```python
from build123d import *

# Parameters (mm, degrees)
BOSS_EXTRUDE1_DEPTH   = 50
BOSS_EXTRUDE1_2_DEPTH = 50
SKETCH3_W             = 160
SKETCH3_H             = 200
BOSS_EXTRUDE2_DEPTH   = 10
FILLET1_R             = 5


with BuildPart() as part:
    # Sketch2 → Boss-Extrude1 (new body)
    with BuildSketch(Plane.XY):
        with BuildLine():
            Line((-70, 20), (-35.355339059, -14.644660941))
            ThreePointArc((-35.355339059, -14.644660941), (-50, -50), (-35.355339059, -85.355339059))
            Line((-35.355339059, -85.355339059), (-50, -100))
            Line((-50, -100), (-80, -100))
            Line((-80, -100), (-80, 100))
            Line((-80, 100), (-50, 100))
            Line((-50, 100), (-50, 80))
            Line((-50, 80), (-28.161785944, 20))
            Line((-28.161785944, 20), (-70, 20))
        make_face()
    extrude(amount=-BOSS_EXTRUDE1_DEPTH)



with BuildPart() as body_2:
    # Sketch2 → Boss-Extrude1 2 (new body)
    with BuildSketch(Plane.XY):
        with BuildLine():
            Line((70, 20), (35.355339059, -14.644660941))
            ThreePointArc((35.355339059, -14.644660941), (50, -50), (35.355339059, -85.355339059))
            Line((35.355339059, -85.355339059), (50, -100))
            Line((50, -100), (80, -100))
            Line((80, -100), (80, 100))
            Line((80, 100), (50, 100))
            Line((50, 100), (50, 80))
            Line((50, 80), (28.161785944, 20))
            Line((28.161785944, 20), (70, 20))
        make_face()
    extrude(amount=-BOSS_EXTRUDE1_2_DEPTH)


with BuildPart() as part_1:
    add(part.part)

    add(body_2.part)  # Boss-Extrude2 merges body 2
    # Sketch3 → Boss-Extrude2 (add)
    with BuildSketch(Plane(origin=(0, 0, -50), x_dir=(-1, 0, 0), z_dir=(0, 0, -1))):
        Rectangle(SKETCH3_W, SKETCH3_H)
    extrude(amount=BOSS_EXTRUDE2_DEPTH)

    # Fillet1
    fillet1_edges = [part_1.edges().sort_by_distance(p)[0] for p in [
        (-28.161785944, 20, -25),
        (-70, 20, -25),
        (70, 20, -25),
        (28.161785944, 20, -25),
    ]]
    fillet(fillet1_edges, radius=FILLET1_R)


solid = part_1.part
```
Can you work these out from the model? Positions are in its coordinate system, mm. A direction names the side the tool comes from. Coordinates: 2 decimals unless noted, no trailing zeros. Order: outer loops, then holes, each group sorted by start corner. A loop starts at its lowest first (then second) coordinate and runs counter-clockwise, first axis right, second up. Notation, with made-up numbers: (3, 82) - (20, 82) arc R7 cw to (20, 88) - close; hole circle Ø10 at (-27.5, 23). An arc over 180 degrees is marked (long way). Answer in a Markdown table with one row per item.
1. Suppose I cut it at B-B (y = 5). Please give me the cut outline in (x, z).
Reply:
| item | result |
|---|---|
| outline | (-80, -60) - (80, -60) - (80, 0) - (55, 0) - (55, -50) - (-55, -50) - (-55, 0) - (-80, 0) - close |
2. If I drill on line 1 along X through (y, z) = (91, -16); line 2 along X through (y, z) = (18.5, -29.5); line 3 along Z through (x, y) = (37, 91), over which ranges is the centre line in solid material (lowest first)?
Reply:
| item | result |
|---|---|
| line 1 | x = -80 to -50, 50 to 80 |
| line 2 | x = -80 to -61.5, 61.5 to 80 |
| line 3 | z = -60 to -50 |
3. Suppose I cut it at C-C (x = -47). Please give me the cut outline in (y, z), and give its area (3 significant figures).
Reply:
| item | result |
|---|---|
| outline | (-100, -60) - (100, -60) - (100, -50) - (71.76, -50) - (71.76, 0) - (20, 0) - (20, -50) - (-3, -50) - (-3, 0) - (-32.94, 0) - (-32.94, -50) - (-67.06, -50) - (-67.06, 0) - (-97, 0) - (-97, -50) - (-100, -50) - close |
| area | 7,580 mm^2 |
4. For pin 1 (1.5 mm diameter, centred on x = -61.5, y = -52, fed in from +Z); pin 2 (6 mm diameter, centred on x = 41, z = -25, fed in from -Y), each with a flat end and sliding along its axis, tell me the tip position at first contact or that it passes through.
Reply:
| item | result |
|---|---|
| pin 1 | stops at z = 0 |
| pin 2 | stops at y = -94 |
5. For faces 1 (the cylindrical face through (-49.997, -49.45, -24.65)), 2 (the flat face through (-43, -93, -25)), 3 (the flat face through (-80, -1, -30)), 4 (the flat face through (50, 90, -25)), which set-ups out of +Z, -Z, +X, -X, +Y, -Y let a thin tool reach every point of the face, with its end or its side?
Reply:
| item | result |
|---|---|
| face 1 | +Z |
| face 2 | +Z, -Y |
| face 3 | +Z, -Z, -X, +Y, -Y |
| face 4 | +Z, +Y |
6. Suppose I cut it at A-A (z = -41.5). Please give me the cut outline in (x, y).
Reply:
| item | result |
|---|---|
| outline | (-80, -100) - (-50, -100) - (-35.36, -85.36) arc R50 cw to (-35.36, -14.64) - (-61.46, 11.46) arc R5 cw to (-57.93, 20) - (-35.3, 20) arc R5 ccw to (-30.6, 26.71) - (-50, 80) - (-50, 100) - (-80, 100) - close; (30.6, 26.71) arc R5 ccw to (35.3, 20) - (57.93, 20) arc R5 cw to (61.46, 11.46) - (35.36, -14.64) arc R50 cw to (35.36, -85.36) - (50, -100) - (80, -100) - (80, 100) - (50, 100) - (50, 80) - close |
7. If we mould it in two halves opening along Y, with no side actions, what happens to faces 5 (the flat face through (-40.44, 53.73, -24.65)), 6 (the cylindrical face through (62.58, 16.84, -25.35)), 7 (the flat face through (43, -93, -25))? For each: pulls with the +Y half, pulls with the -Y half, needs draft (parallel to the pull), parting line crosses it, or undercut.
Reply:
| item | result |
|---|---|
| face 5 | pulls with the +Y half |
| face 6 | undercut |
| face 7 | pulls with the -Y half |
8. Suppose I cut it at D-D (y = -72.5). Please give me the cut outline in (x, z).
Reply:
| item | result |
|---|---|
| outline | (-80, -60) - (80, -60) - (80, 0) - (44.65, 0) - (44.65, -50) - (-44.65, -50) - (-44.65, 0) - (-80, 0) - close |
